Geometry check sheet. Reference: the model listing, model coordinates, mm. A direction names the side the tool comes from. Round coordinates to 2 decimals unless told otherwise and drop trailing zeros. Write item = value, one per line.
from build123d import *

# Parameters (mm, degrees)
SKETCH1_W           = 107.315
SKETCH1_H           = 139.7
SKETCH1_R           = 1.7272
BOSS_EXTRUDE1_DEPTH = 3.2004
SKETCH2_W           = 12.7
SKETCH2_H           = 25.4
CUT_EXTRUDE1_DEPTH  = 3.2004
FILLET1_R           = 2.54
SKETCH3_W           = 2.54
SKETCH3_H           = 3.81
CUT_EXTRUDE2_DEPTH  = 3.2004


with BuildPart() as part:
    # Sketch1 → Boss-Extrude1 (new body)
    with BuildSketch(Plane(origin=(0, 0, 0), x_dir=(1, 0, 0), z_dir=(0, 1, 0))):
        with Locations((53.6575, 69.85)):
            Rectangle(SKETCH1_W, SKETCH1_H)
        with Locations(Location((10.795, 132.0165, 0), (0, 0, 270))):
            Circle(SKETCH1_R, mode=Mode.SUBTRACT)
        with Locations(Location((96.52, 132.0165, 0), (0, 0, 270))):
            Circle(SKETCH1_R, mode=Mode.SUBTRACT)
        with Locations(Location((96.52, 7.6835, 0), (0, 0, 270))):
            Circle(SKETCH1_R, mode=Mode.SUBTRACT)
        with Locations(Location((10.795, 7.6835, 0), (0, 0, 270))):
            Circle(SKETCH1_R, mode=Mode.SUBTRACT)
    extrude(amount=BOSS_EXTRUDE1_DEPTH)

    # Sketch2 → Cut-Extrude1 (cut)
    with BuildSketch(Plane(origin=(0, 3.2004, 0), x_dir=(1, 0, 0), z_dir=(0, 1, 0))):
        with BuildLine():
            Line((0, 119.38), (0, 93.98))
            ThreePointArc((0, 93.98), (11.036508986, 106.68), (0, 119.38))
        make_face()
        with Locations((22.86, 106.68)):
            Rectangle(SKETCH2_W, SKETCH2_H)
    extrude(amount=-CUT_EXTRUDE1_DEPTH, mode=Mode.SUBTRACT)

    # Fillet1
    fillet1_edges = [part.edges().sort_by_distance(p)[0] for p in [
        (0, 1.6002, -119.38),
        (0, 1.6002, -93.98),
        (0, 1.6002, -139.7),
        (107.315, 1.6002, -139.7),
        (107.315, 1.6002, 0),
        (0, 1.6002, 0),
    ]]
    fillet(fillet1_edges, radius=FILLET1_R)

    # Sketch3 → Cut-Extrude2 (cut)
    with BuildSketch(Plane(origin=(0, 3.2004, 0), x_dir=(1, 0, 0), z_dir=(0, 1, 0))):
        with Locations((92.075, 43.815)):
            Rectangle(SKETCH3_W, SKETCH3_H)
        with Locations((12.7, 95.885)):
            Rectangle(SKETCH3_W, SKETCH3_H)
        with Locations((97.155, 43.815)):
            Rectangle(SKETCH3_W, SKETCH3_H)
        with Locations((97.155, 95.885)):
            Rectangle(SKETCH3_W, SKETCH3_H)
        with Locations((92.075, 95.885)):
            Rectangle(SKETCH3_W, SKETCH3_H)
        with Locations((10.16, 43.815)):
            Rectangle(SKETCH3_W, SKETCH3_H)
        with Locations((15.24, 43.815)):
            Rectangle(SKETCH3_W, SKETCH3_H)
    extrude(amount=-CUT_EXTRUDE2_DEPTH, mode=Mode.SUBTRACT)


solid = part.part
(1) Tool access check on faces 1 (the flat face through (53, 0, -71)), 2 (the flat face through (93.345, 2, -96)). Record the directions out of +Z, -Z, +X, -X, +Y, -Y that give a thin tool (end or side, any length) a straight path to the whole face; none if there is none.
Result set:
face_1 = +Z, -Z, +X, -X, -Y
face_2 = +Y, -Y
(2) Release check for a two-part mould opening along X. For faces 3 (the flat face through (107.315, 2, -69)), 4 (the flat face through (23, 2, -93.98)), 5 (the flat face through (53, 2, -139.7)) record: released by +X, released by -X, zero draft, split by the parting line, or undercut.
Result set:
face_3 = released by +X
face_4 = undercut
face_5 = zero draft
(3) Sectioned sample at A-A on y = 0.9. State how many separate pieces and enclosed holes the cut face has, then the cut area to 3 significant figures.
Result set:
separate_pieces = 1
enclosed_holes = 12
area = 14,300 mm2
(4) Depth check by flat-ended pin: pin 1 Ø1.6 at (y, z) = (2.5, -96) entering from -X. Enter the tip coordinate at first touch or a pass-through.
Result set:
pin_1 = 3.93
(5) Material ranges on line 1 along Z through (x, y) = (96.52, 2.55); line 2 along Z through (x, y) = (28, 0.2); line 3 along Z through (x, y) = (16, 1.4), recorded low to high. Write a range as from..to.
Result set:
line_1 = -139.7..-133.74, -130.29..-97.79, -93.98..-45.72, -41.91..-9.41, -5.96..0
line_2 = -139.7..-119.38, -93.98..0
line_3 = -139.7..-45.72, -41.91..0
